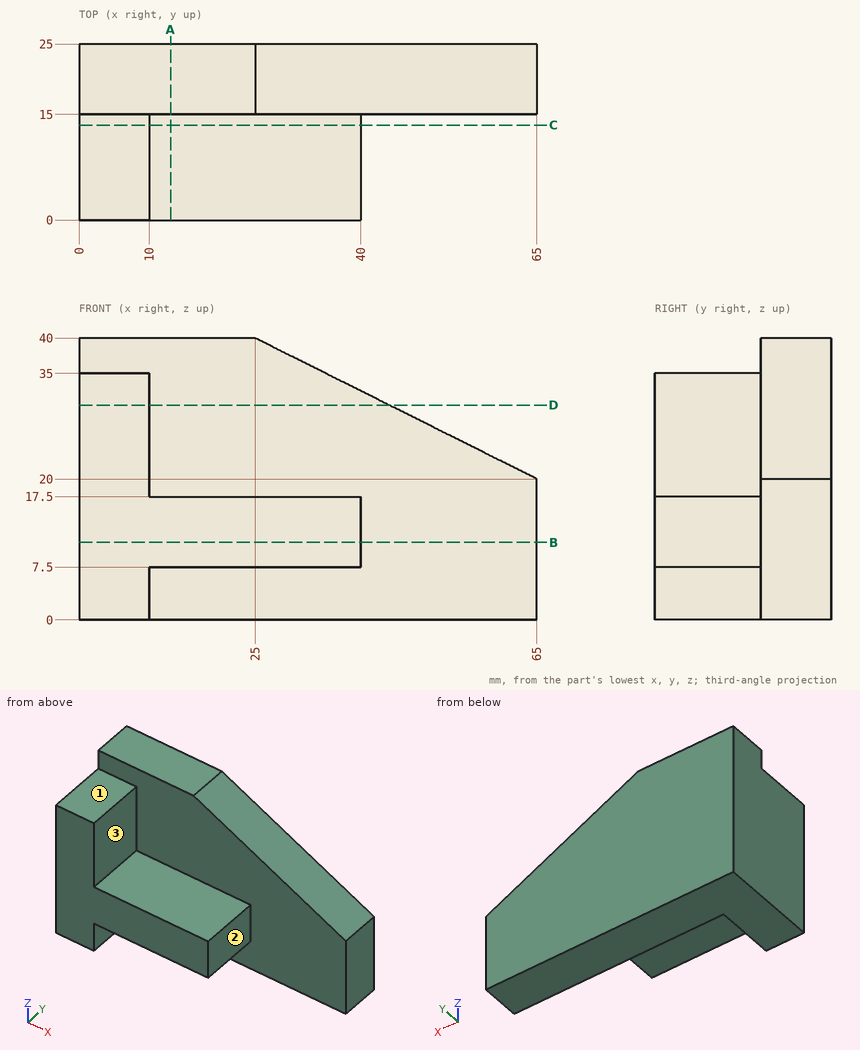
Answer from the drawing. Dimensions are ordinates in mm from the lowest x, y and z of the part. A direction names the side the tool comes from. Give positions to 0.01 mm unless a question says otherwise; leave off trailing zeros. Order: outer loops, then holes, each group sorted by start corner. A loop starts at its lowest first (then second) coordinate and runs counter-clockwise, first axis right, second up. Notation, with made-up numbers: (58.5, -34) -> (113.5, -34) arc R10 ccw to (113.5, -26) -> close; hole circle Ø9 at (88, 71). An arc over 180 degrees is marked (long way). Answer as a JSON object with one key per item and string values. Group by question number.
1. A tool of negligible diameter and unlimited length cuts with its end or side. For the marked faces 1, 2 and 3, from which of +Z, -Z, +X, -X, +Y, -Y can it reach the whole face along a straight path? Write none if from no direction.
2. Section C-C on y = 13.5 is taken. Determine the outline of the cut face in (x, z).
3. Section D-D on z = 30.5 is taken. Determine the outline of the cut face in (x, y).
4. Consider line 1 along Y through (x, z) = (47, 7); line 2 along Z through (x, y) = (7.5, 12); line 3 along Z through (x, y) = (12, 7.75). Determine where each line is inside the solid, lowest interval first. Write a range as [from, to].
5. Flat-ended cylindrical pins translate along their axes: pin 1 Ø10 at (y, z) = (19.5, 29.5) entering from +X; pin 2 Ø2 at (y, z) = (12.5, 5.5) entering from +X; pin 3 Ø8 at (y, z) = (8, 5.5) entering from -X; pin 4 Ø3 at (y, z) = (8, 15) entering from +X. Find the tip coordinate at first contact, or state that the pin passes through.
6. Section A-A on x = 13 is taken. Determine the outline of the cut face in (y, z).
7. Section B-B on z = 11 is taken. Determine the outline of the cut face in (x, y), plus the area to 3 significant figures.
Result sheet:
{
 "1": {"face 1": "+Z, +X, -X, -Y", "face 2": "+Z, -Z, +X, -Y", "face 3": "+Z, +X, -Y"},
 "2": {"outline": "(0, 0) -> (10, 0) -> (10, 7.5) -> (40, 7.5) -> (40, 17.5) -> (10, 17.5) -> (10, 35) -> (0, 35) -> close"},
 "3": {"outline": "(0, 0) -> (10, 0) -> (10, 15) -> (44, 15) -> (44, 25) -> (0, 25) -> close"},
 "4": {"line 1": "y = [15, 25]", "line 2": "z = [0, 35]", "line 3": "z = [7.5, 17.5]"},
 "5": {"pin 1": "stops at x = 56", "pin 2": "stops at x = 10", "pin 3": "stops at x = 0", "pin 4": "stops at x = 40"},
 "6": {"outline": "(0, 7.5) -> (15, 7.5) -> (15, 0) -> (25, 0) -> (25, 40) -> (15, 40) -> (15, 17.5) -> (0, 17.5) -> close"},
 "7": {"outline": "(0, 0) -> (40, 0) -> (40, 15) -> (65, 15) -> (65, 25) -> (0, 25) -> close", "area": "1,250 mm^2"}
}
